Autodesk Fusion 360 part; units mm, degrees
box "PrimitivaParallelepipedo1" add length 400 width 500 height 30 placed x (0, 1, 0) y (-1, 0, 0) z (0, 0, 1) at (500, 0, 0)
sketch "Schizzo2" plane through (0, 0, 0) normal (0, 0, -1) x (1, 0, 0)
  line L0 (0, -400) -> (500, -400)
  line L1 (500, -400) -> (500, 0)
  line L2 (500, 0) -> (0, 0)
  line L3 (0, 0) -> (0, -400)
  line L4 (0, 0) -> (40, 0)
  line L5 (40, 0) -> (40, -40)
  line L6 (40, -40) -> (0, -40)
  line L7 (0, -40) -> (0, 0)
  line L8 (500, 0) -> (460, 0)
  line L9 (460, 0) -> (460, -40)
  line L10 (460, -40) -> (500, -40)
  line L11 (500, -40) -> (500, 0)
  line L12 (500, -400) -> (460, -400)
  line L13 (460, -400) -> (460, -360)
  line L14 (460, -360) -> (500, -360)
  line L15 (500, -360) -> (500, -400)
  line L16 (0, -400) -> (40, -400)
  line L17 (40, -400) -> (40, -360)
  line L18 (40, -360) -> (0, -360)
  line L19 (0, -360) -> (0, -400)
  dimension "d6" = 40
  dimension "d7" = 40
  dimension "d8" = 40
  dimension "d9" = 40
extrude "Estrusione1" add sketch "Schizzo2" along normal blind 1070 contours L0 L3 L16 L17 L18 L19 | L0 L1 L12 L13 L14 L15 | L2 L3 L4 L5 L6 L7 | L1 L2 L8 L9 L10 L11
component "Component" placed x (1, 0, 0) y (0, 1, 0) z (0, 0, 1) at (0, 0, 0)
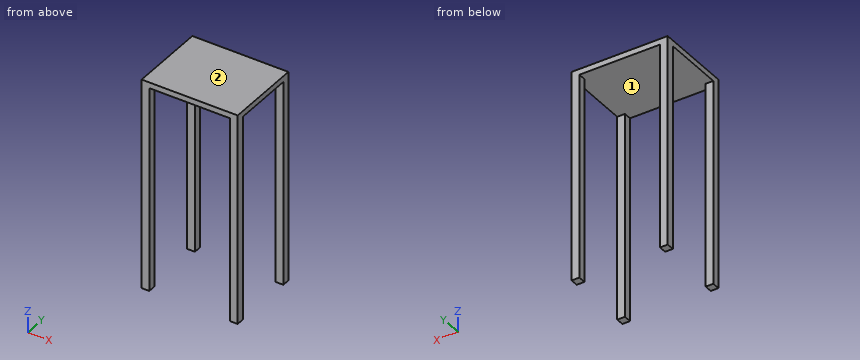
Geometry: final body of the model. Coordinates: model frame, mm. Face numbers are marked on the shaded views. Give positions to 0.01 mm unless a question says otherwise; leave off trailing zeros. Write each loop counter-clockwise with the first axis right and the second up, starting at its lowest first coordinate (ties: lowest second). Pieces come first, ordered by that corner, then holes. Notation, with made-up numbers: (-18.75, 62) -> (25.25, 62) arc R24 ccw to (25.25, 99) -> close; hole circle Ø1 at (-9.5, -20). An arc over 180 degrees is marked (long way). Answer in a Markdown table with one row per item.
(1) Pin query (flat end, axial travel): pin 1 (20 mm diameter, centred on x = 17.5, z = -760, fed in from -Y); pin 2 (2 mm diameter, centred on x = 268, y = 294, fed in from -Z). Return the tip coordinate at first contact, or that it passes through.
Answers below:
| item | result |
|---|---|
| pin 1 | y = 0 |
| pin 2 | z = 0 |
(2) Ray query, line 1 along X through (y, z) = (378, -627); line 2 along Y through (x, z) = (476, -350); line 3 along Z through (x, y) = (263, 144). Return the intervals inside material, ascending. Write a range as [from, to].
Answers below:
| item | result |
|---|---|
| line 1 | [0, 40], [460, 500] |
| line 2 | [0, 40], [360, 400] |
| line 3 | [0, 30] |
(3) Section query B-B on y = 65.5. Return loops of the section in (x, z), then the cut area to 3 significant figures.
Answers below:
| item | result |
|---|---|
| outline | (0, 0) -> (500, 0) -> (500, 30) -> (0, 30) -> close |
| area | 15,000 mm^2 |
(4) Draft query along Y for the marked faces 1 and 2. Return one class per face: +Y half, -Y half, draft (parallel to the pull), parting line (faces both ways), or undercut.
Answers below:
| item | result |
|---|---|
| face 1 | undercut |
| face 2 | draft |
(5) Section query A-A on z = -608. Return loops of the section in (x, y), then the cut area to 3 significant figures.
Answers below:
| item | result |
|---|---|
| outline | (0, 0) -> (40, 0) -> (40, 40) -> (0, 40) -> close; (0, 360) -> (40, 360) -> (40, 400) -> (0, 400) -> close; (460, 0) -> (500, 0) -> (500, 40) -> (460, 40) -> close; (460, 360) -> (500, 360) -> (500, 400) -> (460, 400) -> close |
| area | 6,400 mm^2 |
(6) Section query C-C on x = 447.5. Return loops of the section in (y, z), then the cut area to 3 significant figures.
Answers below:
| item | result |
|---|---|
| outline | (0, 0) -> (400, 0) -> (400, 30) -> (0, 30) -> close |
| area | 12,000 mm^2 |
